Work out the finished part from the listing and answer in its coordinate system (mm). A direction names the side the tool comes from. Coordinates: 2 decimals unless noted, no trailing zeros. Order: outer loops, then holes, each group sorted by start corner. A loop starts at its lowest first (then second) coordinate and runs counter-clockwise, first axis right, second up. Notation, with made-up numbers: (4.5, -22.5) -> (51.5, -22.5) arc R17 cw to (51.5, -8.5) -> close; hole circle Ø2 at (68, -9.75). An arc over 180 degrees is marked (long way). Write item = value, one per line. Start each with the question number.
Q1. Flat-ended cylindrical pins translate along their axes: pin 1 (5 mm diameter, centred on x = -8, y = 4, fed in from +Z); pin 2 (5 mm diameter, centred on y = 4.5, z = -30, fed in from +X); pin 3 (8 mm diameter, centred on x = -5.5, y = 15, fed in from +Z); pin 4 (5 mm diameter, centred on x = 24.5, z = 67, fed in from +Y). Find the tip coordinate at first contact, or state that the pin passes through.
Q2. The part is cut by section B-B, the plane x = -57.5. Determine the outline of the cut face in (y, z).
Q3. Straight lines are drawn through the part: L1, parallel to Y at x = 9, z = -38; L2, parallel to Y at x = 0, z = 0.5; L3, parallel to Y at x = 18, z = -2. For each, find the intervals that lie inside material, in ascending order. Write a range as from..to.
Q4. Which of the six approach directions +Z, -Z, +X, -X, +Y, -Y give full straight-line access (tool end or side, diameter ignored) to faces 4 (the flat face through (-3, 15, 2.5)), 5 (the flat face through (-37.76, 1.23, 64.2))?
Q5. For a pull along X with two mould halves and no side action, classify faces 1 (the flat face through (-36.72, 1.23, -64.8)), 2 (the flat face through (-3, 15, -2.5)), 3 (the flat face through (37.76, 1.23, -64.2)) as +X half, -X half, draft (parallel to the pull), parting line (faces both ways), or undercut.
Q6. The part is cut by section A-A, the plane z = 10.5. Determine the outline of the cut face in (x, y).
```python
from build123d import *

# Parameters (mm, degrees)
BOSS_EXTRUDE1_DEPTH = 2.5
BOSS_EXTRUDE3_DEPTH = 2.5


with BuildPart() as part:
    # Sketch1 → Boss-Extrude1 (new body)
    with BuildSketch(Plane(origin=(0, 0, 0), x_dir=(1, 0, 0), z_dir=(0, 1, 0))):
        Polygon((74.478184725, 43), (0, 86), (-74.478184725, 43), (-74.478184725, -43), (0, -86), (74.478184725, -43), align=None)
    extrude(amount=BOSS_EXTRUDE1_DEPTH)

    # Sketch3 → Boss-Extrude3 (add, symmetric)
    with BuildSketch(Plane.XY):
        with BuildLine():
            Line((-34.925061785, 2.5), (-33.920058448, 2.5))
            add(Edge.make_bspline(
                [(-33.920058448, 2.5), (-33.917714333, 2.524136942), (-33.913611653, 2.566166439), (-33.866227824, 3.047358518), (-33.766675223, 3.968656997), (-33.543636065, 5.697492998), (-33.208094305, 7.727036524), (-32.732470915, 9.857688537), (-32.007597516, 12.3221702), (-30.947827565, 14.726109244), (-29.496843491, 16.656599478), (-27.918808177, 17.817788786), (-25.584089516, 18.616023277), (-22.027089573, 18.448365095), (-16.980597414, 17.01454632), (-11.504417112, 15.301442536), (-6.727145071, 14.453209419), (-2.889367791, 14.698102091), (0.821978206, 15.488717654), (5.270865061, 17.204085784), (10.310286951, 19.65834123), (15.042453427, 21.768085831), (18.653774649, 22.640567877), (21.300542559, 22.524752908), (23.196966016, 21.975950032), (25.06481994, 20.867848988), (26.936162582, 19.06478675), (28.798725849, 16.441516786), (30.32418762, 13.488682834), (31.519963625, 10.621236271), (32.402488107, 8.209159025), (33.126607206, 5.965942013), (33.665257214, 4.140301082), (33.931776285, 3.187716336), (34.072246391, 2.672840674), (34.101906516, 2.563465), (34.119055988, 2.5)],
                knots=[0, 0, 0, 0, 0.000400295, 0.000667158, 0.0078125, 0.015625, 0.03125, 0.046875, 0.0625, 0.09375, 0.125, 0.15625, 0.1875, 0.25, 0.3125, 0.375, 0.4375, 0.46875, 0.5, 0.5625, 0.625, 0.6875, 0.75, 0.78125, 0.8125, 0.84375, 0.875, 0.90625, 0.9375, 0.953125, 0.96875, 0.984375, 0.9921875, 0.998375544, 0.999025327, 1, 1, 1, 1], degree=3))
            Line((34.119055988, 2.5), (35.074938215, 2.5))
            add(Edge.make_bspline(
                [(-34.925061785, 2.5), (-32.150541188, 30.388634665), (-0.320997251, -3.695090393), (25.079154745, 39.838944932), (35.074938215, 2.5)],
                knots=[0, 0, 0, 0, 0.444258071, 1, 1, 1, 1], degree=3))
        make_face()
    extrude(amount=BOSS_EXTRUDE3_DEPTH, both=True)


solid = part.part
```
Model answer:
q1.pin_1 = 82.54
q1.pin_2 = 74.48
q1.pin_3 = 2.5
q1.pin_4 = 2.5
q2.outline = (0, -52.8) -> (2.5, -52.8) -> (2.5, 52.8) -> (0, 52.8) -> close
q3.L1 = 0..2.5
q3.L2 = 0..2.5, 15.37..16.22
q3.L3 = 0..2.5, 22.4..23.18
q4.face_4 = +Z, +X, -X, +Y
q4.face_5 = +Z, -X, +Y, -Y
q5.face_1 = -X half
q5.face_2 = draft
q5.face_3 = +X half
q6.outline = (-74.48, 0) -> (74.48, 0) -> (74.48, 2.5) -> (-74.48, 2.5) -> close
